Input: part model. Units: mm. Frame: model coordinates. A direction names the side the tool comes from. Round coordinates to 2 decimals unless told otherwise and drop trailing zeros. Order: outer loops, then holes, each group sorted by start corner. A loop starts at its lowest first (then second) coordinate and runs counter-clockwise, first axis right, second up. Notation, with made-up numbers: (71.5, -28.5) -> (106.5, -28.5) arc R27 ccw to (106.5, -11.5) -> close; hole circle Ø6 at (-8, 5.25). An arc over 180 degrees is marked (long way). Use a Markdown table: item, result.
from build123d import *

# Parameters (mm, degrees)
SKETCH_1_W          = 15
SKETCH_1_H          = 15
SKETCH_1_W_2        = 12
SKETCH_1_H_2        = 12
EXTRUDE_1_DEPTH     = 500
SKETCH_2_R          = 2.25
CUT_EXTRUDE_1_DEPTH = 25
SKETCH_3_R          = 2.25
CUT_EXTRUDE_2_DEPTH = 25
SKETCH_4_R          = 2.25
CUT_EXTRUDE_3_DEPTH = 20
SKETCH_5_R          = 5
CUT_EXTRUDE_4_DEPTH = 10
SKETCH_6_R          = 5
CUT_EXTRUDE_5_DEPTH = 10


with BuildPart() as part:
    # ｽｹｯﾁ1 → ﾎﾞｽ - 押し出し1 (new body)
    with BuildSketch(Plane.XY):
        Rectangle(SKETCH_1_W, SKETCH_1_H)
        Rectangle(SKETCH_1_W_2, SKETCH_1_H_2, mode=Mode.SUBTRACT)
    extrude(amount=EXTRUDE_1_DEPTH)

    # ｽｹｯﾁ2 → ｶｯﾄ - 押し出し1 (cut)
    with BuildSketch(Plane(origin=(7.5, 0, 0), x_dir=(0, 0, -1), z_dir=(1, 0, 0))):
        with Locations((-492.5, 0)):
            Circle(SKETCH_2_R)
        with Locations((-7.5, 0)):
            Circle(SKETCH_2_R)
        with Locations((-317.5, 0)):
            Circle(SKETCH_2_R)
        with Locations((-182.5, 0)):
            Circle(SKETCH_2_R)
    extrude(amount=-CUT_EXTRUDE_1_DEPTH, mode=Mode.SUBTRACT)

    # ｽｹｯﾁ3 → ｶｯﾄ - 押し出し2 (cut)
    with BuildSketch(Plane(origin=(0, 7.5, 0), x_dir=(1, 0, 0), z_dir=(0, 1, 0))):
        with Locations((0, -22.5)):
            Circle(SKETCH_3_R)
        with Locations((0, -477.5)):
            Circle(SKETCH_3_R)
        with Locations((0, -37.5)):
            Circle(SKETCH_3_R)
        with Locations((0, -462.5)):
            Circle(SKETCH_3_R)
        with Locations((0, -67.5)):
            Circle(SKETCH_3_R)
        with Locations((0, -432.5)):
            Circle(SKETCH_3_R)
    extrude(amount=-CUT_EXTRUDE_2_DEPTH, mode=Mode.SUBTRACT)

    # ｽｹｯﾁ4 → ｶｯﾄ - 押し出し3 (cut)
    with BuildSketch(Plane(origin=(0, -7.5, 0), x_dir=(-1, 0, 0), z_dir=(0, -1, 0))):
        with Locations((0, -390)):
            Circle(SKETCH_4_R)
        with Locations((0, -330)):
            Circle(SKETCH_4_R)
        with Locations((0, -110)):
            Circle(SKETCH_4_R)
        with Locations((0, -170)):
            Circle(SKETCH_4_R)
    extrude(amount=-CUT_EXTRUDE_3_DEPTH, mode=Mode.SUBTRACT)

    # ｽｹｯﾁ5 → ｶｯﾄ - 押し出し4 (cut)
    with BuildSketch(Plane(origin=(0, 7.5, 0), x_dir=(1, 0, 0), z_dir=(0, 1, 0))):
        with Locations((0, -22.5)):
            Circle(SKETCH_5_R)
        with Locations((0, -477.5)):
            Circle(SKETCH_5_R)
        with Locations((0, -390)):
            Circle(SKETCH_5_R)
        with Locations((0, -330)):
            Circle(SKETCH_5_R)
        with Locations((0, -110)):
            Circle(SKETCH_5_R)
        with Locations((0, -170)):
            Circle(SKETCH_5_R)
    extrude(amount=-CUT_EXTRUDE_4_DEPTH, mode=Mode.SUBTRACT)

    # ｽｹｯﾁ6 → ｶｯﾄ - 押し出し5 (cut)
    with BuildSketch(Plane(origin=(7.5, 0, 0), x_dir=(0, 0, -1), z_dir=(1, 0, 0))):
        with Locations((-492.5, 0)):
            Circle(SKETCH_6_R)
        with Locations((-317.5, 0)):
            Circle(SKETCH_6_R)
        with Locations((-182.5, 0)):
            Circle(SKETCH_6_R)
        with Locations((-7.5, 0)):
            Circle(SKETCH_6_R)
    extrude(amount=-CUT_EXTRUDE_5_DEPTH, mode=Mode.SUBTRACT)


solid = part.part
1) Set-up query: faces 1 (the face through (0, 6, 246)), 2 (the face through (6.76, 1.5, 487.73)), 3 (the face through (-0.651, 6.76, 472.543)). Return all of +Z, -Z, +X, -X, +Y, -Y with unobstructed straight access to the full face (end or side cutting, diameter ignored); none if empty.
Answer key:
| item | result |
|---|---|
| face 1 | +Z, -Z |
| face 2 | +X |
| face 3 | +Y |
2) Cut plane B-B on y = 0. State how many separate pieces and enclosed holes the cut face has, and give its area (3 significant figures).
Answer key:
| item | result |
|---|---|
| separate pieces | 10 |
| enclosed holes | 0 |
| area | 1,410 mm^2 |
3) Contact query for flat-ended pins moving along their axis: P1, Ø6, axis at x = 0, z = 330, coming from the +Y side; P2, Ø9, axis at y = 0, z = 317.5, coming from the +X side. Output: stop coordinate, or through.
Answer key:
| item | result |
|---|---|
| P1 | stops at y = -6 |
| P2 | stops at x = -6 |
4) Draft query along Z for faces 4 (the face through (6.76, 0.22, 187.495)), 5 (the face through (-7, 0, 500)), 6 (the face through (6, 0, 246)). Return one class per face: released by +Z, released by -Z, zero draft, split by the parting line, or undercut.
Answer key:
| item | result |
|---|---|
| face 4 | undercut |
| face 5 | released by +Z |
| face 6 | zero draft |
5) Cut plane A-A on z = 224. Return loops of the section in (x, y).
Answer key:
| item | result |
|---|---|
| outline | (-7.5, -7.5) -> (7.5, -7.5) -> (7.5, 7.5) -> (-7.5, 7.5) -> close; hole (-6, -6) -> (6, -6) -> (6, 6) -> (-6, 6) -> close |
6) Ray query, probe 1 along Y at (x, z) = (3, 245.5); probe 2 along X at (y, z) = (6.8, 330). Return the intervals inside material, ascending.
Answer key:
| item | result |
|---|---|
| probe 1 | y = -7.5 to -6, 6 to 7.5 |
| probe 2 | x = -7.5 to -5, 5 to 7.5 |
